```python
from build123d import *

# Parameters (mm, degrees)
TAP_DRILL_FOR_M3_TAP1_D          = 2.5
SKETCH6_W                        = 1.25
SKETCH6_H                        = 12.7
TAP_DRILL_FOR_M3_TAP2_AT_2_COUNT = 2
TAP_DRILL_FOR_M3_TAP2_AT_2_PITCH = 4.6


with BuildPart() as part:
    # Sketch1 → Revolve1 (revolve)
    with BuildSketch(Plane.XY, mode=Mode.PRIVATE) as revolve1_sk:
        Polygon((3, 0), (3, 9.2), (6, 9.2), (6, 5), (12.7, 5), (12.7, 0), align=None)
    revolve(revolve1_sk.sketch.rotate(Axis((0, 0, 0), (0, 1, 0)), 90), axis=Axis((0, 0, 0), (0, 1, 0)))

    # Tap Drill for M3 Tap1 (through all)
    with Locations(Plane(origin=(0, 5, 0), x_dir=(1, 0, 0), z_dir=(0, 1, 0))):
        with Locations((-9.5, 0), (-4.75, 8.227241336), (4.75, 8.227241336), (9.5, 0), (4.75, -8.227241336), (-4.75, -8.227241336)):
            Hole(TAP_DRILL_FOR_M3_TAP1_D / 2)

    # Sketch6 → Tap Drill for M3 Tap2 (revolve, cut)
    with BuildSketch(Plane(origin=(0, 2.5, 0), x_dir=(0, 1, 0), z_dir=(1, 0, 0))):
        with Locations((0.625, 6.35)):
            Rectangle(SKETCH6_W, SKETCH6_H)
    tap_drill_for_m3_tap2 = revolve(axis=Axis((0, 2.5, -6.35), (0, 0, 1)), mode=Mode.SUBTRACT)

    # Tap Drill for M3 Tap2 at 2: Tap Drill for M3 Tap2 ×2
    with Locations(*[(0, i * TAP_DRILL_FOR_M3_TAP2_AT_2_PITCH, 0) for i in range(1, TAP_DRILL_FOR_M3_TAP2_AT_2_COUNT)]):
        add(tap_drill_for_m3_tap2, mode=Mode.SUBTRACT)


solid = part.part
```
Can you work these out from the model? Positions are in its coordinate system, mm. A direction names the side the tool comes from. Round coordinates to 2 decimals unless told otherwise and drop trailing zeros. Loops run counter-clockwise (first coordinate to the right, second up) from the corner with the lowest first, then second, coordinate; pieces in that order, holes last. Notation, with made-up numbers: M 82,-33 L 112,-33 A24 ccw 112,4 Z; hole C 32.5,19 d11. An arc over 180 degrees is marked long. Answer in a Markdown table with one row per item.
1. I'm going to push flat-ended pins straight in: pin 1 Ø3 at (x, z) = (-9.5, 0) entering from +Y; pin 2 Ø3 at (x, y) = (3.5, 3) entering from -Z; pin 3 Ø1.5 at (y, z) = (6.5, -2.5) entering from +X. Where does each tip first touch, or does it pass through?
Established:
| item | result |
|---|---|
| pin 1 | y = 5 |
| pin 2 | z = -12.54 |
| pin 3 | x = 5.74 |
2. If we section it at B-B, the plane x = 0: Please give me the cut outline in (y, z).
Established:
| item | result |
|---|---|
| outline | M 0,-12.7 L 5,-12.7 L 5,-6 L 9.2,-6 L 9.2,-3 L 0,-3 Z; M 0,3 L 1.25,3 L 1.25,12.7 L 0,12.7 Z; M 3.75,3 L 5.85,3 L 5.85,6 L 5,6 L 5,12.7 L 3.75,12.7 Z; M 8.35,3 L 9.2,3 L 9.2,6 L 8.35,6 Z |
3. Please list where these lines run through material, in increasing order: line 1 (Y direction, x = 0, z = 10.75); line 2 (Z direction, x = -4.75, y = 2.75); line 3 (Z direction, x = 5.5, y = 2.5). Write a range as from..to.
Established:
| item | result |
|---|---|
| line 1 | 0..1.25, 3.75..5 |
| line 2 | -11.78..-9.48, -6.98..6.98, 9.48..11.78 |
| line 3 | -11.45..-9.23, -7.23..7.23, 9.23..11.45 |
4. If we section it at A-A, the plane z = 0: Please give me the cut outline in (x, y).
Established:
| item | result |
|---|---|
| outline | M -12.7,0 L -10.75,0 L -10.75,5 L -12.7,5 Z; M -8.25,0 L -3,0 L -3,9.2 L -6,9.2 L -6,5 L -8.25,5 Z; M 3,0 L 8.25,0 L 8.25,5 L 6,5 L 6,9.2 L 3,9.2 Z; M 10.75,0 L 12.7,0 L 12.7,5 L 10.75,5 Z |
5. Thinking about a two-plate mould opening in X: for faces 4 (the face through (-8.25, 2.47, -0.05)), 5 (the face through (-1.802, 7.071, -5.723)), 6 (the face through (3, 0, -3)), which applies, pulls with the +X half, pulls with the -X half, needs draft (parallel to the pull), parting line crosses it, or undercut?
Established:
| item | result |
|---|---|
| face 4 | undercut |
| face 5 | parting line crosses it |
| face 6 | needs draft |
6. If we section it at C-C, the plane y = 0.5: Please give me the cut outline in (x, z), plus the area to 3 significant figures.
Established:
| item | result |
|---|---|
| outline | C 0,0 d25.4; hole C -9.5,0 d2.5; hole C -4.75,-8.23 d2.5; hole C -4.75,8.23 d2.5; hole C 0,0 d6; hole C 4.75,-8.23 d2.5; hole C 4.75,8.23 d2.5; hole C 9.5,0 d2.5 |
| area | 449 mm² |
7. On a 3-axis mill with a long thin cutter (end or side, diameter ignored), from which of +Z, -Z, +X, -X, +Y, -Y can I reach the whole of each face in a straight line? I mean faces 1 (the face through (-0.38, 3.69, 7.78)), 2 (the face through (5.021, 2.465, 9.448)), 3 (the face through (5.5, 5, -3)). Say none if no direction works.
Established:
| item | result |
|---|---|
| face 1 | +Z |
| face 2 | +Y, -Y |
| face 3 | +Y |
8. If we section it at D-D, the plane x = 9.5: Please give me the cut outline in (y, z), plus the area to 3 significant figures.
Established:
| item | result |
|---|---|
| outline | M 0,-8.43 L 5,-8.43 L 5,-1.25 L 0,-1.25 Z; M 0,1.25 L 5,1.25 L 5,8.43 L 0,8.43 Z |
| area | 71.8 mm² |
